from build123d import *

# Parameters (mm, degrees)
F2_R     = 15
F2_R_2   = 7.5
F3_DEPTH = 5
F2_R_3   = 3.3
F4_DEPTH = 19
F2_R_4   = 6
F5_DEPTH = 28.8
F6_DEPTH = 1
F7_SIZE  = 2


with BuildPart() as f1:
    # F0 (on Front) → F1 (revolve)
    with BuildSketch(Plane.XZ):
        with BuildLine():
            Line((0, -19.3), (0, 0))
            Line((0, 0), (-68, 0))
            Line((-68, 0), (-68, -6.3))
            ThreePointArc((-68, -6.3), (-63.606602, -16.906602), (-53, -21.3))
            Line((-53, -21.3), (-42, -21.3))
            Line((-42, -21.3), (-42, -19.3))
            Line((-42, -19.3), (0, -19.3))
        make_face()
    revolve(axis=Axis((0, 0, -9.65), (0, 0, -1)))

    # F2 (on face) → F3 (join)
    with BuildSketch(Plane.XY):
        with Locations((-25, 40)):
            Circle(F2_R)
        with Locations((-25, 40)):
            Circle(F2_R_2, mode=Mode.SUBTRACT)
        with Locations((25, 40)):
            Circle(F2_R)
        with Locations((25, 40)):
            Circle(F2_R_2, mode=Mode.SUBTRACT)
        with Locations((25, 0)):
            Circle(F2_R)
        with Locations((25, 0)):
            Circle(F2_R_2, mode=Mode.SUBTRACT)
        with Locations((-25, 0)):
            Circle(F2_R)
        with Locations((-25, 0)):
            Circle(F2_R_2, mode=Mode.SUBTRACT)
    extrude(amount=F3_DEPTH)

    # F2 (on face) → F4 (cut)
    with BuildSketch(Plane.XY):
        with Locations((-25, 40)):
            Circle(F2_R_2)
        with Locations((25, 40)):
            Circle(F2_R_2)
        with Locations((25, 0)):
            Circle(F2_R_2)
        with Locations((-25, 0)):
            Circle(F2_R_2)
        with Locations((-25, -40)):
            Circle(F2_R_3)
        with Locations((25, -40)):
            Circle(F2_R_3)
    extrude(amount=-F4_DEPTH, mode=Mode.SUBTRACT)

    # F2 (on face) → F5 (join)
    with BuildSketch(Plane.XY):
        with Locations((-25, -40)):
            Circle(F2_R_4)
        with Locations((-25, -40)):
            Circle(F2_R_3, mode=Mode.SUBTRACT)
        with Locations((25, -40)):
            Circle(F2_R_4)
        with Locations((25, -40)):
            Circle(F2_R_3, mode=Mode.SUBTRACT)
    extrude(amount=F5_DEPTH)

    # F2 (on face) → F6 (join)
    with BuildSketch(Plane.XY):
        with Locations((-25, -40)):
            Circle(F2_R)
        with Locations((-25, -40)):
            Circle(F2_R_4, mode=Mode.SUBTRACT)
        with Locations((25, -40)):
            Circle(F2_R)
        with Locations((25, -40)):
            Circle(F2_R_4, mode=Mode.SUBTRACT)
    extrude(amount=F6_DEPTH)

    # F7
    f7_edges = [f1.edges().sort_by_distance(p)[0] for p in [
        (-32.5, 40, 5),
        (17.5, 40, 5),
        (17.5, 0, 5),
        (-32.5, 0, 5),
        (-31, -40, 28.8),
        (19, -40, 28.8),
    ]]
    chamfer(f7_edges, length=F7_SIZE)


solid = f1.part
Work out the finished part from the listing and answer in its coordinate system (mm). A direction names the side the tool comes from. Give positions to 0.01 mm unless a question says otherwise; leave off trailing zeros. Write each loop counter-clockwise with the first axis right and the second up, starting at its lowest first coordinate (ties: lowest second). Pieces come first, ordered by that corner, then holes.
Q1. The part is cut by section A-A on z = -3. Give the vertices of the cut face in (x, y), and give its area (3 significant figures).
Answer:
outline: circle Ø136 at (0, 0); hole circle Ø15 at (-25, 0); hole circle Ø15 at (-25, 40); hole circle Ø6.6 at (-25, -40); hole circle Ø15 at (25, 0); hole circle Ø15 at (25, 40); hole circle Ø6.6 at (25, -40)
area: 13,800 mm2
Q2. A tool of negligible diameter and unlimited length cuts with its end or side. For faces 1 (the face through (25, 40, -19)), 2 (the face through (32, 28, -21.3)), 3 (the face through (1, 1, -19.3)), from which of +Z, -Z, +X, -X, +Y, -Y can it reach the whole face along a straight path? Write none if from no direction.
Answer:
face 1: +Z
face 2: -Z, +X, -X, +Y, -Y
face 3: -Z
Q3. Given pin 1 (2 mm diameter, centred on x = 14, y = 34.5, fed in from -Z); pin 2 (4 mm diameter, centred on x = 29.5, z = -10, fed in from +Y); pin 3 (3 mm diameter, centred on x = 19, z = -16, fed in from +Y), each flat-ended and moving along its own axis, determine where each tip first touches the part or whether it passes through.
Answer:
pin 1: stops at z = -19.3
pin 2: stops at y = 61.81
pin 3: stops at y = 62.84
Q4. The part is cut by section D-D on z = 17. Give the vertices of the cut face in (x, y), and give its area (3 significant figures).
Answer:
outline: circle Ø12 at (-25, -40); circle Ø12 at (25, -40); hole circle Ø6.6 at (-25, -40); hole circle Ø6.6 at (25, -40)
area: 158 mm2
Q5. Straight lines are drawn through the part: L1, parallel to X at y = 46, z = -5.5; L2, parallel to Y at x = 25, z = -13; L3, parallel to Y at x = 25, z = -8. For each, find the intervals that lie inside material, in ascending order.
Answer:
L1: x = -50.08 to -29.5, -20.5 to 20.5, 29.5 to 50.08
L2: y = -61.54 to -43.3, -36.7 to -7.5, 7.5 to 32.5, 47.5 to 61.54
L3: y = -63.13 to -43.3, -36.7 to -7.5, 7.5 to 32.5, 47.5 to 63.13
Q6. The part is cut by section C-C on x = 0. Give the vertices of the cut face in (y, z), and give its area (3 significant figures).
Answer:
outline: (-68, -6.3) arc R15 ccw to (-53, -21.3) - (-42, -21.3) - (-42, -19.3) - (42, -19.3) - (42, -21.3) - (53, -21.3) arc R15 ccw to (68, -6.3) - (68, 0) - (-68, 0) - close
area: 2,630 mm2
Q7. For a pull along X with two mould halves and no side action, classify faces 4 (the face through (-25, 40, -19)), 5 (the face through (23.37, 32.68, -8.15)), 6 (the face through (-15, 40, 5)) as released by +X, released by -X, zero draft, split by the parting line, or undercut.
Answer:
face 4: undercut
face 5: undercut
face 6: zero draft
